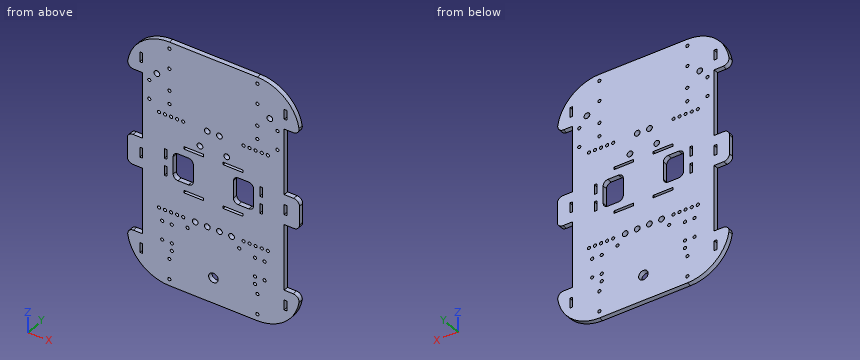
```python
from build123d import *

# Parameters (mm, degrees)
SKETCH2_W           = 2.7
SKETCH2_H           = 10.51
SKETCH2_H_2         = 10.666666666
BOSS_EXTRUDE4_DEPTH = 5
SKETCH5_R           = 1.65
SKETCH5_R_2         = 3
SKETCH5_R_3         = 5
SKETCH5_W           = 20.48
SKETCH5_H           = 2.7
SKETCH5_W_2         = 2.7
SKETCH5_H_2         = 10.42
CUT_EXTRUDE1_DEPTH  = 6


with BuildPart() as part:
    # Sketch2 → Boss-Extrude4 (new body)
    with BuildSketch(Plane(origin=(0, 0, 0), x_dir=(1, 0, 0), z_dir=(0, 1, 0))):
        with BuildLine():
            Line((46, -130), (-46, -130))
            ThreePointArc((-46, -130), (-74.550970119, -119.478980051), (-89.448061775, -92.947368421))
            ThreePointArc((-89.448061775, -92.947368421), (-88.08864154, -88.106685893), (-83.523326079, -86))
            Line((-83.523326079, -86), (-74, -86))
            Line((-74, -86), (-74, -16))
            Line((-74, -16), (-84, -16))
            ThreePointArc((-84, -16), (-88.242640687, -14.242640687), (-90, -10))
            Line((-90, -10), (-90, 10))
            ThreePointArc((-90, 10), (-88.242640687, 14.242640687), (-84, 16))
            Line((-84, 16), (-74, 16))
            Line((-74, 16), (-74, 86))
            Line((-74, 86), (-83.523326079, 86))
            ThreePointArc((-83.523326079, 86), (-88.08864154, 88.106685893), (-89.448061775, 92.947368421))
            ThreePointArc((-89.448061775, 92.947368421), (-74.550970119, 119.478980051), (-46, 130))
            Line((-46, 130), (46, 130))
            ThreePointArc((46, 130), (74.550970119, 119.478980051), (89.448061775, 92.947368421))
            ThreePointArc((89.448061775, 92.947368421), (88.08864154, 88.106685893), (83.523326079, 86))
            Line((83.523326079, 86), (74, 86))
            Line((74, 86), (74, 16))
            Line((74, 16), (84, 16))
            ThreePointArc((84, 16), (88.242640687, 14.242640687), (90, 10))
            Line((90, 10), (90, -10))
            ThreePointArc((90, -10), (88.242640687, -14.242640687), (84, -16))
            Line((84, -16), (74, -16))
            Line((74, -16), (74, -86))
            Line((74, -86), (83.523326079, -86))
            ThreePointArc((83.523326079, -86), (88.08864154, -88.106685893), (89.448061775, -92.947368421))
            ThreePointArc((89.448061775, -92.947368421), (74.550970119, -119.478980051), (46, -130))
        make_face()
        with Locations((-75.35, 101.765)):
            Rectangle(SKETCH2_W, SKETCH2_H, mode=Mode.SUBTRACT)
        with Locations((75.35, 101.765)):
            Rectangle(SKETCH2_W, SKETCH2_H, mode=Mode.SUBTRACT)
        with Locations((75.35, -101.765)):
            Rectangle(SKETCH2_W, SKETCH2_H, mode=Mode.SUBTRACT)
        with Locations((-75.35, -101.765)):
            Rectangle(SKETCH2_W, SKETCH2_H, mode=Mode.SUBTRACT)
        with Locations((-75.35, 0)):
            Rectangle(SKETCH2_W, SKETCH2_H_2, mode=Mode.SUBTRACT)
        with Locations((75.35, 0)):
            Rectangle(SKETCH2_W, SKETCH2_H_2, mode=Mode.SUBTRACT)
    extrude(amount=BOSS_EXTRUDE4_DEPTH)

    # Sketch5 → Cut-Extrude1 (cut, through all)
    with BuildSketch(Plane(origin=(0, 5, 0), x_dir=(1, 0, 0), z_dir=(0, 1, 0))):
        with Locations((-56.9, -51)):
            Circle(SKETCH5_R)
        with Locations((-50.55, -51)):
            Circle(SKETCH5_R)
        with Locations((-44.2, -51)):
            Circle(SKETCH5_R)
        with Locations((-37.85, -51)):
            Circle(SKETCH5_R)
        with Locations((-31.5, -51)):
            Circle(SKETCH5_R)
        with Locations((31.5, -51)):
            Circle(SKETCH5_R)
        with Locations((37.85, -51)):
            Circle(SKETCH5_R)
        with Locations((44.2, -51)):
            Circle(SKETCH5_R)
        with Locations((50.55, -51)):
            Circle(SKETCH5_R)
        with Locations((56.9, -51)):
            Circle(SKETCH5_R)
        with Locations((56.9, 51)):
            Circle(SKETCH5_R)
        with Locations((50.55, 51)):
            Circle(SKETCH5_R)
        with Locations((44.2, 51)):
            Circle(SKETCH5_R)
        with Locations((37.85, 51)):
            Circle(SKETCH5_R)
        with Locations((31.5, 51)):
            Circle(SKETCH5_R)
        with Locations((-31.5, 51)):
            Circle(SKETCH5_R)
        with Locations((-37.85, 51)):
            Circle(SKETCH5_R)
        with Locations((-44.2, 51)):
            Circle(SKETCH5_R)
        with Locations((-50.55, 51)):
            Circle(SKETCH5_R)
        with Locations((-56.9, 51)):
            Circle(SKETCH5_R)
        with Locations((-14, -32)):
            Circle(SKETCH5_R_2)
        with Locations((14, -32)):
            Circle(SKETCH5_R_2)
        with Locations((19, 51)):
            Circle(SKETCH5_R_2)
        with Locations((-19, 51)):
            Circle(SKETCH5_R_2)
        with Locations((-53.5, 83.83)):
            Circle(SKETCH5_R)
        with Locations((-53.5, 63.83)):
            Circle(SKETCH5_R)
        with Locations((-43.5, 63.83)):
            Circle(SKETCH5_R)
        with Locations((-43.5, 83.83)):
            Circle(SKETCH5_R)
        with Locations((43.5, 63.83)):
            Circle(SKETCH5_R)
        with Locations((53.5, 63.83)):
            Circle(SKETCH5_R)
        with Locations((43.5, 83.83)):
            Circle(SKETCH5_R)
        with Locations((53.5, 83.83)):
            Circle(SKETCH5_R)
        with Locations((-46, 123)):
            Circle(SKETCH5_R)
        with Locations((-46, 101.5)):
            Circle(SKETCH5_R)
        with Locations((46, 101.5)):
            Circle(SKETCH5_R)
        with Locations((46, 123)):
            Circle(SKETCH5_R)
        with Locations((-67, -60.960027583)):
            Circle(SKETCH5_R)
        with Locations((-45.897115189, -63.923125828)):
            Circle(SKETCH5_R)
        with Locations((-67, -81.039972417)):
            Circle(SKETCH5_R)
        with Locations((-45.897115189, -78.156819007)):
            Circle(SKETCH5_R)
        with Locations((45.897115189, -63.923125828)):
            Circle(SKETCH5_R)
        with Locations((45.897115189, -78.156819007)):
            Circle(SKETCH5_R)
        with Locations((67, -81.039972417)):
            Circle(SKETCH5_R)
        with Locations((67, -60.960027583)):
            Circle(SKETCH5_R)
        with Locations((46, -123)):
            Circle(SKETCH5_R)
        with Locations((46, -101.5)):
            Circle(SKETCH5_R)
        with Locations((-46, -101.5)):
            Circle(SKETCH5_R)
        with Locations((-46, -123)):
            Circle(SKETCH5_R)
        with Locations((-27, 60.5)):
            Circle(SKETCH5_R)
        with Locations((27, 60.5)):
            Circle(SKETCH5_R)
        with Locations((-43.5, 91.83)):
            Circle(SKETCH5_R)
        with Locations((43.5, 91.83)):
            Circle(SKETCH5_R)
        with Locations((-6.333333333, 51)):
            Circle(SKETCH5_R_2)
        with Locations((6.333333333, 51)):
            Circle(SKETCH5_R_2)
        with Locations((0, 103)):
            Circle(SKETCH5_R_3)
        with Locations((59, -91.08)):
            Circle(SKETCH5_R_2)
        with Locations((-59, -91.08)):
            Circle(SKETCH5_R_2)
        with Locations((-6.333333333, -51)):
            Circle(SKETCH5_R_2)
        with Locations((6.333333333, -51)):
            Circle(SKETCH5_R_2)
        with Locations((20.48, -23.35)):
            Rectangle(SKETCH5_W, SKETCH5_H)
        with Locations((-20.48, -23.35)):
            Rectangle(SKETCH5_W, SKETCH5_H)
        with Locations((20.48, 23.35)):
            Rectangle(SKETCH5_W, SKETCH5_H)
        with Locations((-20.48, 23.35)):
            Rectangle(SKETCH5_W, SKETCH5_H)
        with Locations((49.85, -9.07)):
            Rectangle(SKETCH5_W_2, SKETCH5_H_2)
        with Locations((49.85, 9.07)):
            Rectangle(SKETCH5_W_2, SKETCH5_H_2)
        with Locations((-49.85, 9.07)):
            Rectangle(SKETCH5_W_2, SKETCH5_H_2)
        with Locations((-49.85, -9.07)):
            Rectangle(SKETCH5_W_2, SKETCH5_H_2)
        with BuildLine():
            Line((37.006010734, 14.28), (26.003005367, 14.28))
            ThreePointArc((26.003005367, 14.28), (22.467471461, 12.815533906), (21.003005367, 9.28))
            Line((21.003005367, 9.28), (21.003005367, -7.14))
            Line((21.003005367, -7.14), (21.003005367, -9.28))
            ThreePointArc((21.003005367, -9.28), (22.467471461, -12.815533906), (26.003005367, -14.28))
            Line((26.003005367, -14.28), (37.006010734, -14.28))
            ThreePointArc((37.006010734, -14.28), (40.54154464, -12.815533906), (42.006010734, -9.28))
            Line((42.006010734, -9.28), (42.006010734, 9.28))
            ThreePointArc((42.006010734, 9.28), (40.54154464, 12.815533906), (37.006010734, 14.28))
        make_face()
        with BuildLine():
            Line((-42.006010734, 9.28), (-42.006010734, -9.28))
            ThreePointArc((-42.006010734, -9.28), (-40.54154464, -12.815533906), (-37.006010734, -14.28))
            Line((-37.006010734, -14.28), (-26.003005367, -14.28))
            ThreePointArc((-26.003005367, -14.28), (-22.467471461, -12.815533906), (-21.003005367, -9.28))
            Line((-21.003005367, -9.28), (-21.003005367, 9.28))
            ThreePointArc((-21.003005367, 9.28), (-22.467471461, 12.815533906), (-26.003005367, 14.28))
            Line((-26.003005367, 14.28), (-37.006010734, 14.28))
            ThreePointArc((-37.006010734, 14.28), (-40.54154464, 12.815533906), (-42.006010734, 9.28))
        make_face()
    extrude(amount=-CUT_EXTRUDE1_DEPTH, mode=Mode.SUBTRACT)


solid = part.part
```
Source: CAD feature listing. Evaluate the final solid. Frame: model axes, mm. Round coordinates to 2 decimals unless told otherwise and drop trailing zeros. Loops run counter-clockwise (first coordinate to the right, second up) from the corner with the lowest first, then second, coordinate; pieces in that order, holes last. Notation, with made-up numbers: M 37.25,-18.5 L 94.25,-18.5 A21 cw 94.25,11.5 Z; hole C -32,42 d8. An arc over 180 degrees is marked long. Use a Markdown table: item, result. Add a question column.
1. Cut plane B-B, the plane y = 2.15. State how many separate pieces and enclosed holes the cut face has, and give its area (3 significant figures).
2. Cut plane A-A, the plane z = -1. Output: boundary loops of the cut face in (x, y).
3. Contact query for flat-ended pins moving along their axis: pin 1 (1.5 mm diameter, centred on y = 4, z = -62.5, fed in from +X); pin 2 (3 mm diameter, centred on x = 53.5, z = -83.83, fed in from +Y); pin 3 (1.3 mm diameter, centred on x = 75, y = 3, fed in from -Z); pin 4 (1.4 mm diameter, centred on x = 49.5, y = 1.5, fed in from -Z). Output: stop coordinate, or through.
4. Ray query, line 1 along X through (y, z) = (2.4, 32); line 2 along Z through (x, y) = (-14, 2.25); line 3 along Z through (x, y) = (-31.5, 3.15). Return the intervals inside material, ascending. Write a range as [from, to].
Solution:
| question | item | result |
|---|---|---|
| 1 | separate pieces | 1 |
| 1 | enclosed holes | 75 |
| 1 | area | 38,200 mm2 |
| 2 | outline | M -90,0 L -76.7,0 L -76.7,5 L -90,5 Z; M -74,0 L -42.01,0 L -42.01,5 L -74,5 Z; M -21,0 L 21,0 L 21,5 L -21,5 Z; M 42.01,0 L 74,0 L 74,5 L 42.01,5 Z; M 76.7,0 L 90,0 L 90,5 L 76.7,5 Z |
| 3 | pin 1 | stops at x = 74 |
| 3 | pin 2 | passes through |
| 3 | pin 3 | stops at z = -119.65 |
| 3 | pin 4 | stops at z = -129.91 |
| 4 | line 1 | x = [-74, -17], [-11, 11], [17, 74] |
| 4 | line 2 | z = [-130, -24.7], [-22, 22], [24.7, 29], [35, 130] |
| 4 | line 3 | z = [-130, -52.65], [-49.35, -14.28], [14.28, 49.35], [52.65, 130] |
